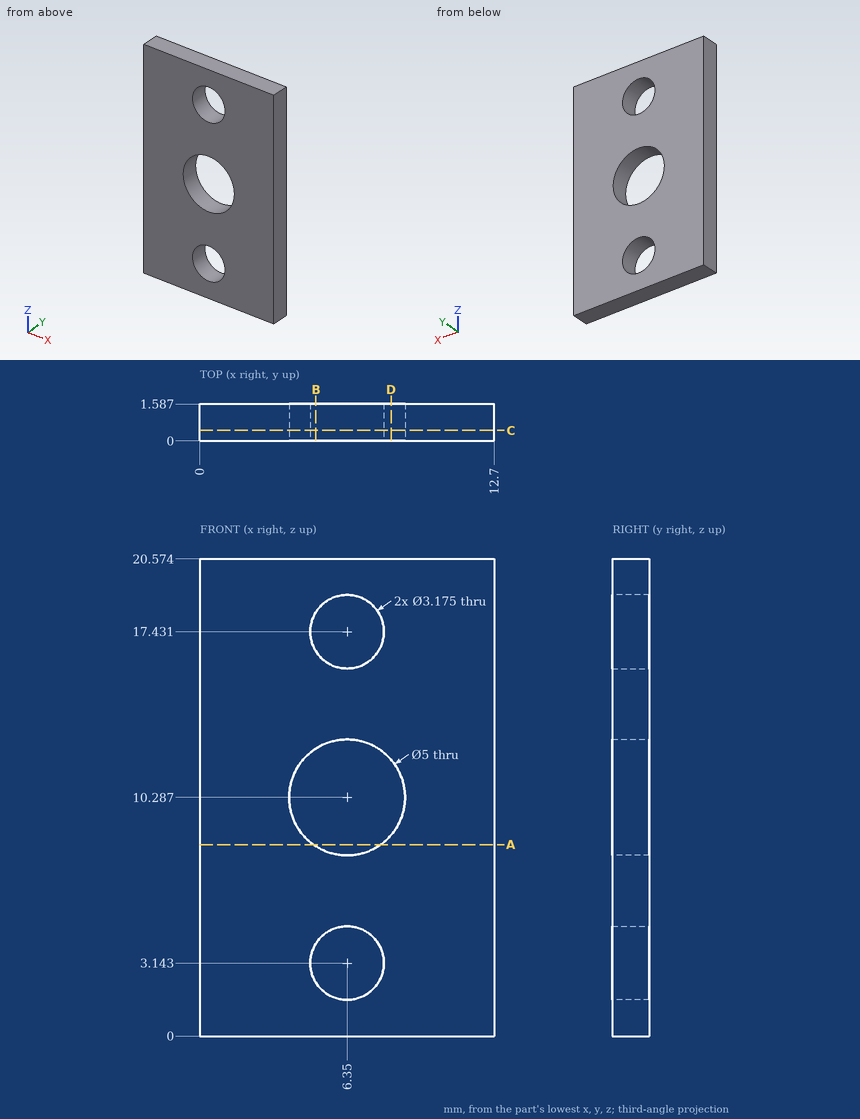
Drawing for the job (mm, zero at the part's lowest x, y, z). Round coordinates to 2 decimals unless told otherwise and drop trailing zeros. Write each loop counter-clockwise with the first axis right and the second up, starting at its lowest first coordinate (ties: lowest second). Pieces come first, ordered by that corner, then holes. Notation, with made-up numbers: M 53.5,-11.75 L 90.5,-11.75 A14 ccw 90.5,-0.75 Z; hole C 12.5,89 d9. An arc over 180 degrees is marked long. Answer as a JSON object with one key per item and string values. Group by question number.
(1) Cut at C-C (y = 0.45). Give the number of separate pieces and of enclosed holes in the cut face, and give its area (3 significant figures).
(2) Cut at B-B (x = 5). Give the cut face in (y, z) (1 decimal).
(3) Drill centre lines: L1, parallel to Z at x = 6.35, y = 1 (1 decimal); L2, parallel to Z at x = 5.75, y = 1.35 (1 decimal); L3, parallel to X at y = 0.1, z = 16 (1 decimal). Where is each one in solid material? Low to high.
(4) Cut at A-A (z = 8.25). Give the cut face in (x, y).
(5) Cut at D-D (x = 8.25). Give the cut face in (y, z) (1 decimal).
(6) Flat gauge pin, fed straight in: pin 1 (2 mm diameter, centred on x = 5, z = 9.5, fed in from -Y). Where does the tip first touch, or does it go through?
Responses:
{
 "1": {"separate pieces": "1", "enclosed holes": "3", "area": "226 mm2"},
 "2": {"outline": "M 0,0 L 1.6,0 L 1.6,2.3 L 0,2.3 Z; M 0,4 L 1.6,4 L 1.6,8.2 L 0,8.2 Z; M 0,12.4 L 1.6,12.4 L 1.6,16.6 L 0,16.6 Z; M 0,18.3 L 1.6,18.3 L 1.6,20.6 L 0,20.6 Z"},
 "3": {"L1": "z = 0 to 1.6, 4.7 to 7.8, 12.8 to 15.8, 19 to 20.6", "L2": "z = 0 to 1.7, 4.6 to 7.9, 12.7 to 16, 18.9 to 20.6", "L3": "x = 0 to 5.7, 7 to 12.7"},
 "4": {"outline": "M 0,0 L 4.9,0 L 4.9,1.59 L 0,1.59 Z; M 7.8,0 L 12.7,0 L 12.7,1.59 L 7.8,1.59 Z"},
 "5": {"outline": "M 0,0 L 1.6,0 L 1.6,8.7 L 0,8.7 Z; M 0,11.9 L 1.6,11.9 L 1.6,20.6 L 0,20.6 Z"},
 "6": {"pin 1": "stops at y = 0"}
}
